Part model, mm, in its own coordinate system. A direction names the side the tool comes from. Give positions to 0.01 mm unless a question says otherwise; leave off trailing zeros. Write each loop counter-clockwise with the first axis right and the second up, starting at its lowest first coordinate (ties: lowest second). Pieces come first, ordered by that corner, then holes.
from build123d import *

# Parameters (mm, degrees)
SKETCH2_W            = 71.5
SKETCH2_H            = 11
BOSS_EXTRUDE2_DEPTH  = 4
SKETCH3_R            = 2
CUT_EXTRUDE1_DEPTH   = 4
SKETCH4_W            = 4
SKETCH4_H            = 4
BOSS_EXTRUDE3_DEPTH  = 11
SKETCH5_W            = 4
SKETCH5_H            = 11
BOSS_EXTRUDE4_DEPTH  = 76
SKETCH7_W            = 75.5
SKETCH7_H            = 11
SKETCH7_R            = 2
BOSS_EXTRUDE5_DEPTH  = 4
SKETCH8_W            = 80
SKETCH8_H            = 11
BOSS_EXTRUDE8_DEPTH  = 4
BOSS_EXTRUDE9_DEPTH  = 25
SKETCH10_R           = 2.5
CUT_EXTRUDE3_DEPTH   = 4
CHAMFER1_SIZE        = 30
SKETCH13_R           = 2
CUT_EXTRUDE4_DEPTH   = 4
BOSS_EXTRUDE10_DEPTH = 4
FILLET1_R            = 10


with BuildPart() as part:
    # Sketch2 → Boss-Extrude2 (new body)
    with BuildSketch(Plane.XY):
        with Locations((35.75, 5.5)):
            Rectangle(SKETCH2_W, SKETCH2_H)
    extrude(amount=BOSS_EXTRUDE2_DEPTH)

    # Sketch3 → Cut-Extrude1 (cut)
    with BuildSketch(Plane.XY.offset(4)):
        with Locations((8, 5.5)):
            Circle(SKETCH3_R)
    extrude(amount=-CUT_EXTRUDE1_DEPTH, mode=Mode.SUBTRACT)

    # Sketch4 → Boss-Extrude3 (add)
    with BuildSketch(Plane(origin=(0, 11, 0), x_dir=(1, 0, 0), z_dir=(0, 1, 0))):
        with Locations((73.5, -2)):
            Rectangle(SKETCH4_W, SKETCH4_H)
    extrude(amount=-BOSS_EXTRUDE3_DEPTH)

    # Sketch5 → Boss-Extrude4 (add)
    with BuildSketch(Plane.XY.offset(4)):
        with Locations((73.5, 5.5)):
            Rectangle(SKETCH5_W, SKETCH5_H)
    extrude(amount=BOSS_EXTRUDE4_DEPTH)



with BuildPart() as body_2:
    # Sketch7 → Boss-Extrude5 (new body)
    with BuildSketch(Plane(origin=(0, 0, 0), x_dir=(-1, 0, 0), z_dir=(0, 0, -1))):
        with Locations((-37.75, 41.5)):
            Rectangle(SKETCH7_W, SKETCH7_H)
        with Locations((-8, 41.5)):
            Circle(SKETCH7_R, mode=Mode.SUBTRACT)
    extrude(amount=-BOSS_EXTRUDE5_DEPTH)

    # Sketch8 → Boss-Extrude8 (add)
    with BuildSketch(Plane(origin=(75.5, 0, 0), x_dir=(0, 0, -1), z_dir=(1, 0, 0))):
        with Locations((-40, 41.5)):
            Rectangle(SKETCH8_W, SKETCH8_H)
    extrude(amount=-BOSS_EXTRUDE8_DEPTH)


with BuildPart() as part_1:
    add(part.part)

    add(body_2.part)  # Boss-Extrude9 merges body 2
    # Sketch9 → Boss-Extrude9 (add)
    with BuildSketch(Plane(origin=(0, 11, 0), x_dir=(1, 0, 0), z_dir=(0, 1, 0))):
        Polygon((75.5, 0), (0, 0), (0, -4), (71.5, -4), (71.5, -80), (75.5, -80), align=None)
    extrude(amount=BOSS_EXTRUDE9_DEPTH)

    # Sketch10 → Cut-Extrude3 (cut)
    with BuildSketch(Plane(origin=(75.5, 0, 0), x_dir=(0, 0, -1), z_dir=(1, 0, 0))):
        with Locations((-48.75, 23.5)):
            Circle(SKETCH10_R)
    extrude(amount=-CUT_EXTRUDE3_DEPTH, mode=Mode.SUBTRACT)

    # Chamfer1
    chamfer1_edges = [part_1.edges().sort_by_distance(p)[0] for p in [
        (75.5, 23.5, 0),
        (71.5, 23.5, 4),
    ]]
    chamfer(chamfer1_edges, length=CHAMFER1_SIZE)

    # Sketch13 → Cut-Extrude4 (cut)
    with BuildSketch(Plane(origin=(75.5, 0, 0), x_dir=(0, 0, -1), z_dir=(1, 0, 0))):
        with Locations((-74.5, 3.5)):
            Circle(SKETCH13_R)
        with Locations((-74.5, 43.5)):
            Circle(SKETCH13_R)
    extrude(amount=-CUT_EXTRUDE4_DEPTH, mode=Mode.SUBTRACT)

    # Sketch14 → Boss-Extrude10 (add)
    with BuildSketch(Plane(origin=(75.5, 0, 0), x_dir=(0, 0, -1), z_dir=(1, 0, 0))):
        Polygon((-82.5, 3.5), (-82.5, 47), (-80, 47), (-80, 0), (-82.5, 0), align=None)
    extrude(amount=-BOSS_EXTRUDE10_DEPTH)

    # Fillet1
    fillet1_edges = [part_1.edges().sort_by_distance(p)[0] for p in [
        (71.5, 23.5, 34),
        (41.5, 23.5, 4),
        (75.5, 23.5, 30),
        (45.5, 23.5, 0),
    ]]
    fillet(fillet1_edges, radius=FILLET1_R)


solid = part_1.part
1) Saw through at B-B (z = 74.5). Write the cut outline in (x, y), and give its area (3 significant figures).
Check result:
outline: (71.5, 0) - (75.5, 0) - (75.5, 1.5) - (71.5, 1.5) - close; (71.5, 5.5) - (75.5, 5.5) - (75.5, 41.5) - (71.5, 41.5) - close; (71.5, 45.5) - (75.5, 45.5) - (75.5, 47) - (71.5, 47) - close
area: 156 mm2
2) 3-axis set-ups, long thin cutter, end or side, ignore diameter. For faces 5 (the flat face through (71.5, 24, 60)), 6 (the flat face through (58, 0, 20)): which of +Z, -Z, +X, -X, +Y, -Y reach the whole face in a straight line?
Check result:
face 5: +Z, -X, +Y, -Y
face 6: +Z, -Z, +X, -X, -Y
3) Saw through at D-D (z = 62). Write the cut outline in (x, y).
Check result:
outline: (71.5, 0) - (75.5, 0) - (75.5, 47) - (71.5, 47) - close
4) Drill centre lines: L1, parallel to Y at x = 73.45, z = 74.5; L2, parallel to Y at x = 8, z = 1; L3, parallel to Z at x = 8.5, y = 18. Where is each one in solid material? Low to high.
Check result:
L1: y = 0 to 1.5, 5.5 to 41.5, 45.5 to 47
L2: y = 0 to 3.5, 7.5 to 39.5, 43.5 to 47
L3: z = 0 to 4
5) Saw through at A-A (x = 8). Write the cut outline in (y, z).
Check result:
outline: (0, 0) - (3.5, 0) - (3.5, 4) - (0, 4) - close; (7.5, 0) - (39.5, 0) - (39.5, 4) - (7.5, 4) - close; (43.5, 0) - (47, 0) - (47, 4) - (43.5, 4) - close
6) Saw through at C-C (y = 23.5). Write the cut outline in (x, z).
Check result:
outline: (0, 0) - (41.36, 0) arc R10 ccw to (48.43, 2.93) - (72.57, 27.07) arc R10 ccw to (75.5, 34.14) - (75.5, 46.25) - (71.5, 46.25) - (71.5, 38.14) arc R10 cw to (68.57, 31.07) - (44.43, 6.93) arc R10 cw to (37.36, 4) - (0, 4) - close; (71.5, 51.25) - (75.5, 51.25) - (75.5, 82.5) - (71.5, 82.5) - close
7) Flat gauge pins, fed straight in: P1, Ø8, axis at y = 18, z = 15, coming from the -X side; P2, Ø1.5, axis at y = 10, z = 21, coming from the +X side; P3, Ø12, axis at x = 11, y = 15.5, coming from the +Z side; P4, Ø3, axis at y = 23.5, z = 48.75, coming from the +X side. Where does each tip first touch, or does it go through?
Check result:
P1: stops at x = 48.5
P2: stops at x = 67.25
P3: stops at z = 4
P4: passes through
8) Mould opens along Z. For faces 1 (the cylindrical face through (73.528, 41.726, 73.577)), 2 (the flat face through (75.5, 24, 58)), 3 (the flat face through (60.7, 23.8, 15.2)), 4 (the flat face through (74, 24, 82.5)) say: +Z half, -Z half, draft (parallel to the pull), parting line (faces both ways), or undercut.
Check result:
face 1: undercut
face 2: draft
face 3: -Z half
face 4: +Z half
